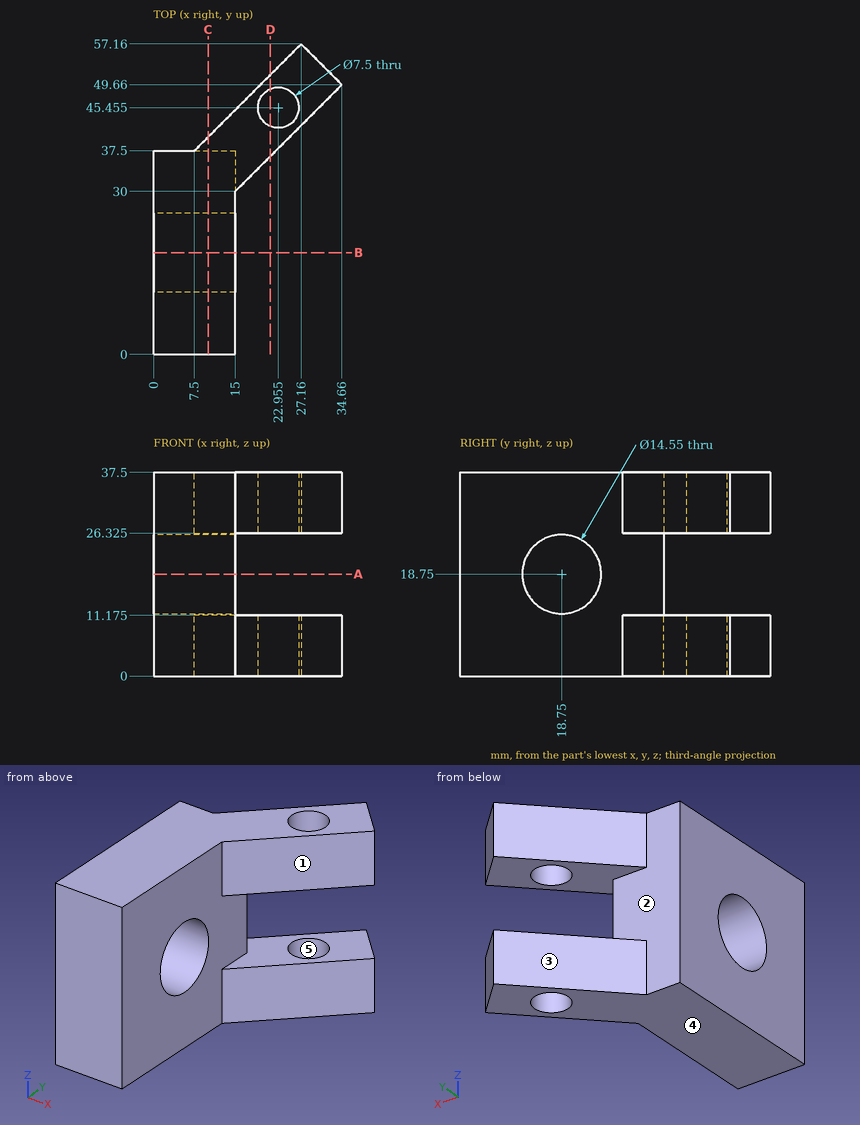
Input: dimensioned drawing with shaded views. Units: mm. Origin: part minimum x, y, z. A direction names the side the tool comes from. Round coordinates to 2 decimals unless told otherwise and drop trailing zeros. Loops run counter-clockwise (first coordinate to the right, second up) from the corner with the lowest first, then second, coordinate; pieces in that order, holes last. Notation, with made-up numbers: (74.25, 60.5) -> (93.25, 60.5) arc R31 cw to (93.25, 95.5) -> close; hole circle Ø5 at (13, 4). An arc over 180 degrees is marked (long way). Answer as a JSON object with one key per item and string values. Group by question number.
Q1. Section query C-C (x = 10). Output: boundary loops of the cut face in (y, z) (3 decimals), plus the area to 3 significant figures.
Q2. Contact query for flat-ended pins moving along their axis: P1, Ø7.5, axis at x = 5, z = 21, coming from the +Y side; P2, Ø12, axis at x = 15.5, z = 22, coming from the +Y side; P3, Ø6, axis at y = 36.5, z = 30.5, coming from the +X side. Output: stop coordinate, or through.
Q3. Section query D-D (x = 21.5). Output: boundary loops of the cut face in (y, z) (3 decimals), plus the area to 3 significant figures.
Q4. Ray query, line 1 (Y direction, x = 7.5, z = 18.75) (3 decimals); line 2 (Z direction, x = 23.5, y = 39) (3 decimals); line 3 (X direction, y = 28.5, z = 21). Return the intervals inside material, ascending. Write a range as from..to.
Q5. Mould query, pull axis Y, two halves, no side actions, for the marked faces 3, 4 and 5. Classes: pulls with the +Y half, pulls with the -Y half, needs draft (parallel to the pull), parting line crosses it, or undercut.
Q6. Access query for the marked faces 1 and 2. Directions: +Z, -Z, +X, -X, +Y, -Y. A direction counts if a zero-diameter tool reaches every point of the face in a straight line with its end or side. Return the directions, or none.
Q7. Section query A-A (z = 18.75). Output: boundary loops of the cut face in (x, y) (3 decimals).
Completed:
{
 "1": {"outline": "(0, 0) -> (40, 0) -> (40, 11.175) -> (37.5, 11.175) -> (37.5, 26.325) -> (40, 26.325) -> (40, 37.5) -> (0, 37.5) -> close; hole circle Ø14.55 at (18.75, 18.75)", "area": "1,300 mm²"},
 "2": {"P1": "y = 37.5", "P2": "y = 49.66", "P3": "x = 24.5"},
 "3": {"outline": "(36.5, 0) -> (41.999, 0) -> (41.999, 11.175) -> (36.5, 11.175) -> close; (36.5, 26.325) -> (41.999, 26.325) -> (41.999, 37.5) -> (36.5, 37.5) -> close; (48.911, 0) -> (51.5, 0) -> (51.5, 11.175) -> (48.911, 11.175) -> close; (48.911, 26.325) -> (51.5, 26.325) -> (51.5, 37.5) -> (48.911, 37.5) -> close", "area": "181 mm²"},
 "4": {"line 1": "0..11.475, 26.025..37.5", "line 2": "0..11.175, 26.325..37.5", "line 3": "0..15"},
 "5": {"face 3": "pulls with the +Y half", "face 4": "needs draft", "face 5": "undercut"},
 "6": {"face 1": "+Z, -Z, +X, -Y", "face 2": "-X, +Y"},
 "7": {"outline": "(0, 0) -> (15, 0) -> (15, 11.475) -> (0, 11.475) -> close; (0, 26.025) -> (15, 26.025) -> (15, 37.5) -> (0, 37.5) -> close"}
}
